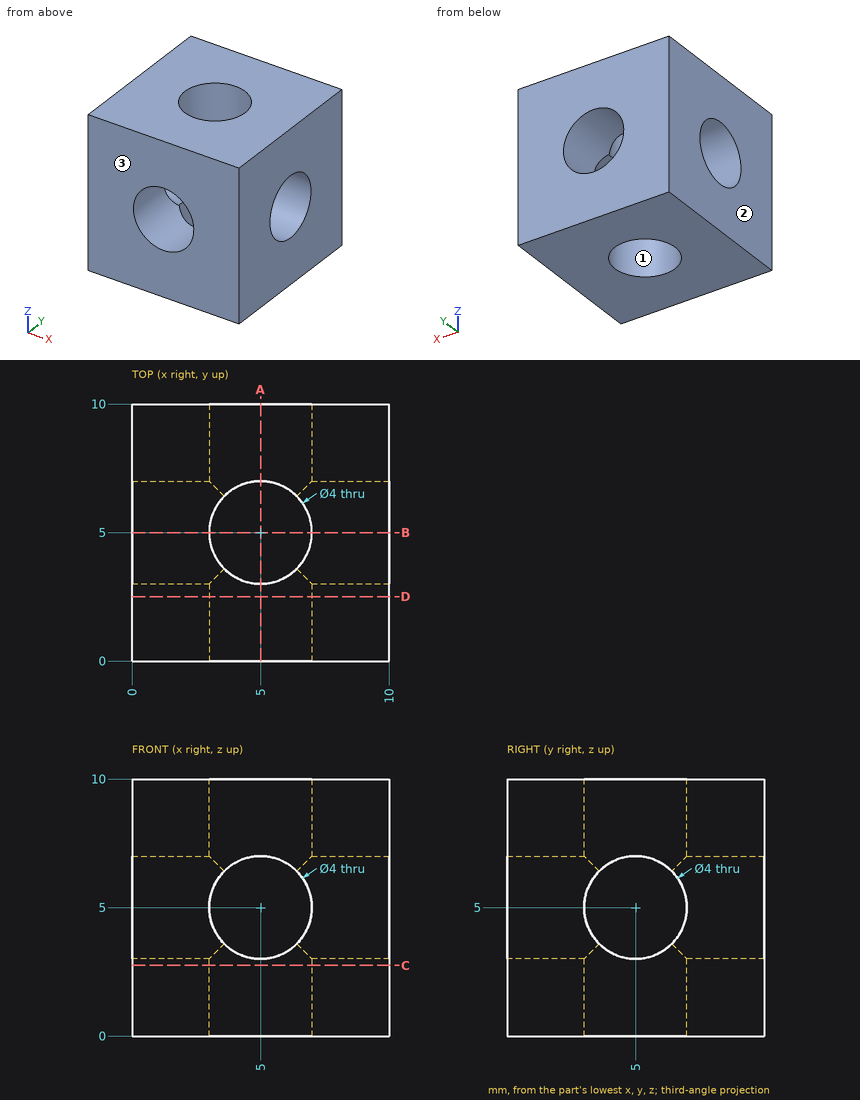
Print and shaded views of the part. All mm, measured from the part's lowest x, y and z. Give positions to 0.01 mm unless a question says otherwise; leave off trailing zeros. Loops run counter-clockwise (first coordinate to the right, second up) from the corner with the lowest first, then second, coordinate; pieces in that order, holes last. Notation, with made-up numbers: (61.5, 5) - (116.5, 5) arc R14 cw to (116.5, 18) - close; hole circle Ø3 at (66.5, -23.5). An arc over 180 degrees is marked (long way). One line per item, written item: value. Start each with the question number.
1. Pull direction X, two halves, no side cores. Call the marked faces 1, 2 and 3: pulls with the +X half, pulls with the -X half, needs draft (parallel to the pull), parting line crosses it, or undercut.
2. Pin check, flat tip, straight feed: pin 1 (3.5 mm diameter, centred on x = 5, z = 5, fed in from -Y). Stop position of the tip, or through.
3. Slice it at A-A (x = 5). List the corners of the cut face in (y, z).
4. Slice it at C-C (z = 2.75). List the corners of the cut face in (x, y).
5. Probe L1, parallel to Z at x = 5, y = 1.55. List the from-to ranges inside material, lowest first. Write a range as from..to.
Solution:
1. face 1: undercut
1. face 2: pulls with the -X half
1. face 3: needs draft
2. pin 1: passes through
3. outline: (0, 0) - (3, 0) - (3, 3) - (0, 3) - close; (0, 7) - (3, 7) - (3, 10) - (0, 10) - close; (7, 0) - (10, 0) - (10, 3) - (7, 3) - close; (7, 7) - (10, 7) - (10, 10) - (7, 10) - close
4. outline: (0, 0) - (10, 0) - (10, 10) - (0, 10) - close; hole circle Ø4 at (5, 5)
5. L1: z = 0..3, 7..10
